from build123d import *


with BuildPart() as f1:
    # F0 (on Right) → F1 (revolve)
    with BuildSketch(Plane.YZ):
        with BuildLine():
            Line((-9.1, 0), (-2.5, 0))
            Line((-2.5, 0), (-2.5, 4))
            Line((-2.5, 4), (-5.1, 6.6))
            Line((-5.1, 6.6), (-5.1, 10))
            Line((-5.1, 10), (-7.1, 10))
            ThreePointArc((-7.1, 10), (-8.514214, 9.414214), (-9.1, 8))
            Line((-9.1, 8), (-9.1, 0))
        make_face()
    revolve(axis=Axis((0, 0, 6.063), (0, 0, 1)))


solid = f1.part
Verification items for the finished model (mm, model axes). A direction names the side the tool comes from. Round coordinates to 2 decimals unless told otherwise and drop trailing zeros. Order: outer loops, then holes, each group sorted by start corner. A loop starts at its lowest first (then second) coordinate and runs counter-clockwise, first axis right, second up.
1. Go/stop test with flat-tipped pins: P1, Ø5, axis at x = -7, z = 8, coming from the +Y side; P2, Ø5, axis at x = 0.5, z = 2, coming from the -Y side; P3, Ø4, axis at x = -6.5, z = 7.5, coming from the -Y side; P4, Ø3, axis at y = -6, z = 2.5, coming from the -X side. Record where each tip stops, or that it passes through.
Final values:
P1: stops at y = 7.91
P2: stops at y = -9.1
P3: stops at y = -7.91
P4: stops at x = -7.91
2. Access from +Z, -Z, +X, -X, +Y, -Y to the whole of each face (thin tool, end or side, straight path). Record for faces 1 (the cylindrical face through (-4.5, -2.4, 8.3)), 2 (the flat face through (2, -5, 10)).
Final values:
face 1: +Z
face 2: +Z, +X, -X, +Y, -Y
3. Release check for a two-part mould opening along Y. For faces 3 (the flat face through (-2, -2, 0)), 4 (the cylindrical face through (-8.884, 1.973, 3.944)), 5 (the conical face through (-2.36, -1.23, 4.16)) record: +Y half, -Y half, draft (parallel to the pull), parting line (faces both ways), or undercut.
Final values:
face 3: draft
face 4: parting line
face 5: undercut
4. Section check A-A on x = 0. Record the cut outline in (y, z), then the cut area to 3 significant figures.
Final values:
outline: (-9.1, 0) - (-2.5, 0) - (-2.5, 4) - (-5.1, 6.6) - (-5.1, 10) - (-7.1, 10) arc R2 ccw to (-9.1, 8) - close; (2.5, 0) - (9.1, 0) - (9.1, 8) arc R2 ccw to (7.1, 10) - (5.1, 10) - (5.1, 6.6) - (2.5, 4) - close
area: 106 mm2
5. Section check C-C on z = 5.5. Record the cut outline in (x, y).
Final values:
outline: circle Ø18.2 at (0, 0); hole circle Ø8 at (0, 0)
6. Section check D-D on z = 3.75. Record the cut outline in (x, y).
Final values:
outline: circle Ø18.2 at (0, 0); hole circle Ø5 at (0, 0)
7. Thickness scan on L1, parallel to X at y = 0, z = 1.65; L2, parallel to Y at x = -0.75, z = 2.25; L3, parallel to X at y = 0, z = 7. Record the ranges inside material, lowest first.
Final values:
L1: x = -9.1 to -2.5, 2.5 to 9.1
L2: y = -9.07 to -2.38, 2.38 to 9.07
L3: x = -9.1 to -5.1, 5.1 to 9.1
